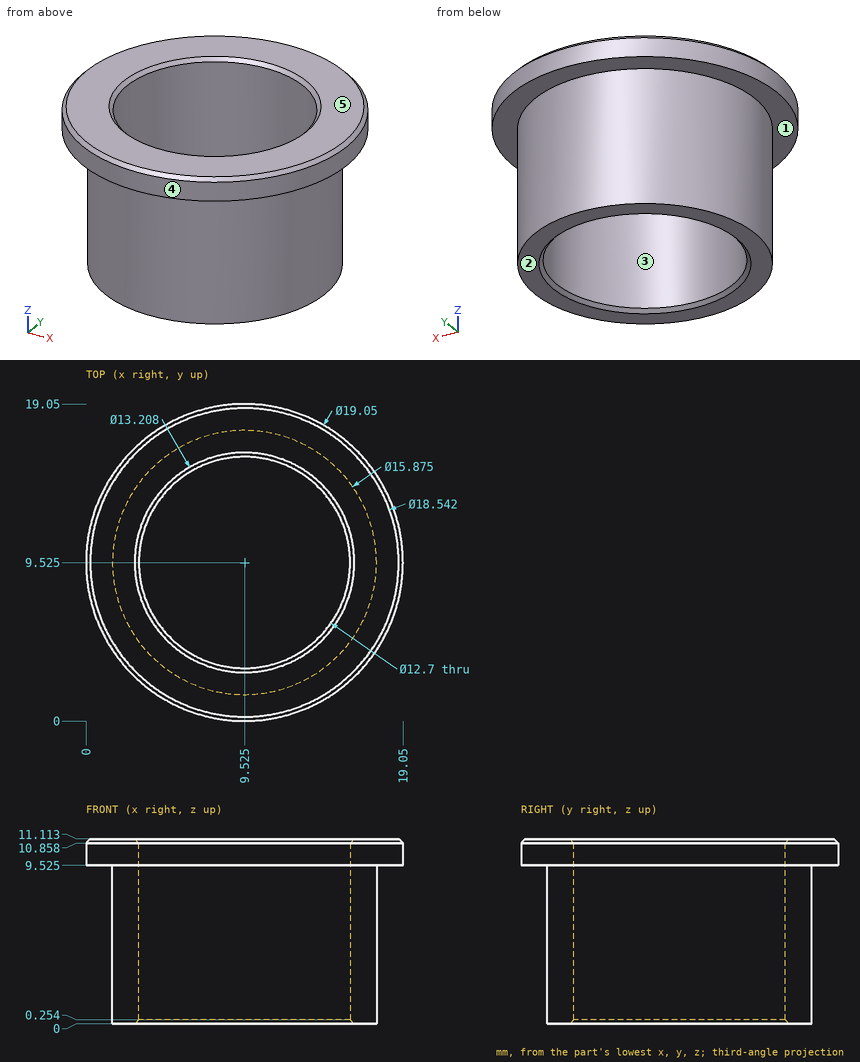
The drawing under review shows one solid part. Ordinate dimensions are in mm from its lowest x, y, z. A direction names the side the tool comes from. Coordinates: 2 decimals unless noted, no trailing zeros. Put each result on its own line as item: value.
1) Insertion check: P1, Ø1, axis at x = 8, z = 8, coming from the +Y side; P2, Ø3, axis at x = 5, y = 9.5, coming from the +Z side; P3, Ø1.5, axis at y = 13.5, z = 3.5, coming from the -X side; P4, Ø3, axis at x = 13, z = 2.5, coming from the +Y side. Each pin has a flat end and moves straight along its axis. Give the tip position at first contact, or say it passes through.
Response values:
P1: stops at y = 17.4
P2: passes through
P3: stops at x = 2.27
P4: stops at y = 17.21
2) Tool access review of the marked faces 1 and 2: name each direction out of +Z, -Z, +X, -X, +Y, -Y from which nothing blocks a thin tool from reaching the whole face with its end or side.
Response values:
face 1: -Z
face 2: -Z, +X, -X, +Y, -Y
3) The part is to be moulded in two halves that separate along Y. For the marked faces 3, 4 and 5, say which applies: released by +Y, released by -Y, zero draft, split by the parting line, or undercut.
Response values:
face 3: undercut
face 4: split by the parting line
face 5: zero draft
4) Wall thickness on L1, parallel to X at y = 9.75, z = 3; L2, parallel to Z at x = 3.5, y = 15 (1 decimal); L3, parallel to X at y = 4.75, z = 8.5 (1 decimal): over which ranges is each line inside the solid? List them lowest first. Write a range as from..to.
Response values:
L1: x = 1.59..3.18, 15.87..17.46
L2: z = 9.5..11.1
L3: x = 3.2..5.3, 13.7..15.9
